Check sheet for the modelled part. Datum: model origin and axes. Units: mm. A direction names the side the tool comes from. Coordinates: 2 decimals unless noted, no trailing zeros. Write each loop counter-clockwise with the first axis right and the second up, starting at its lowest first coordinate (ties: lowest second). Pieces come first, ordered by that corner, then holes. Notation, with made-up numbers: (-10.5, -30) -> (12.5, -30) arc R22 cw to (12.5, 4) -> close; hole circle Ø8 at (-36.75, 9.25). An arc over 180 degrees is marked (long way). One line per item, written item: value. Start each with the question number.
1) Draft check along X on faces 4 (the conical face through (0.621, -0.153, 6.587)), 5 (the flat face through (1, -6, 3)), 6 (the flat face through (3.9, -6, 3)), 7 (the flat face through (4.9, -6, 2)). Enter one of: +X half, -X half, draft (parallel to the pull), parting line (faces both ways), or undercut.
2) Gauge pin test, flat ends, axial feed: P1, Ø2.5, axis at x = 2.5, y = -6, coming from the +Z side; P2, Ø1, axis at x = 3, z = 4.5, coming from the -Y side. Record the tip position at first contact, or that the pin passes through.
3) Sectioned sample at A-A on z = 3. Enter the section's corners in (x, y).
4) Sectioned sample at C-C on x = 2.95. Enter the section's corners in (y, z).
5) Scan lines: line 1 along X through (y, z) = (-5.25, 2.5); line 2 along Z through (x, y) = (1.4, -6.25) (3 decimals); line 3 along Z through (x, y) = (2.8, -11.25). Record each from-to range of solid material in increasing order. Write a range as [from, to].
6) Set-up check for faces 1 (the flat face through (2, -6, 1)), 2 (the flat face through (4.4, -6.4, 5)), 3 (the cylindrical face through (1.21, -6.41, 6.07)): record each of +Z, -Z, +X, -X, +Y, -Y from which the full face is reachable in a straight line by a thin tool's end or side.
7) Sectioned sample at B-B on y = -7.25. Enter the section's corners in (x, z), plus the area to 3 significant figures.
```python
from build123d import *

# Parameters (mm, degrees)
F1_DEPTH     = 13
F2_T1_DEPTH  = 6.0286731952
F2_T3_DEPTH  = 15.0178646599
F2_T5_DEPTH  = 6.9573463904
F2_T7_DEPTH  = 7.0573463904
F2_T10_ANGLE = 67.461453667
F2_T12_ANGLE = 67.461453667


# Not quite as in the source:
# - a fillet or chamfer that OpenCascade refuses, or shapes differently, is made with other operations: its cross-section is extruded or revolved along the edge and cut away or added


with BuildPart() as f1:
    # F0 (on Front) → F1 (new body)
    with BuildSketch(Plane.XZ):
        with BuildLine():
            Line((0, 5), (0, 0))
            Line((0, 0), (4.9, 0))
            Line((4.9, 0), (4.9, 5))
            Line((4.9, 5), (3.9, 5))
            Line((3.9, 5), (3.9, 1))
            Line((3.9, 1), (1, 1))
            Line((1, 1), (1, 5))
            ThreePointArc((1, 5), (1.2914644914, 6.2462400161), (2.1053955316, 7.2339555569))
            Line((2.1053955316, 7.2339555569), (1.4626079219, 8))
            ThreePointArc((1.4626079219, 8), (0.3851271545, 6.6687736465), (0, 5))
        make_face()
    extrude(amount=F1_DEPTH)

    # F2: chamfer of 0.4 on 9 edges, made by hand

    # F2_s2 → F2_t1 (cut)
    with BuildSketch(Plane.XY.offset(-1.0286731952)):
        Polygon((0, -12.6), (0.4, -13), (0, -13), align=None)
        Polygon((0, -0.4), (0.4, 0), (0, 0), align=None)
    extrude(amount=F2_T1_DEPTH, mode=Mode.SUBTRACT)

    # F2_s4 → F2_t3 (cut)
    with BuildSketch(Plane.XZ.offset(-1.00893233)):
        with BuildLine():
            Line((1.8291984844, 6.9931446867), (1.8536490905, 7.5339752825))
            Line((1.8536490905, 7.5339752825), (2.1053955316, 7.2339555569))
            ThreePointArc((2.1053955316, 7.2339555569), (1.9591897538, 7.1144071406), (1.8291984844, 6.9931446867))
        make_face()
    extrude(amount=F2_T3_DEPTH, mode=Mode.SUBTRACT)

    # F2_s6 → F2_t5 (cut)
    with BuildSketch(Plane.YZ.offset(-1.0286731952)):
        Polygon((-0.4, 0), (0, 0.4), (0, 0), align=None)
        Polygon((-12.6, 0), (-13, 0.4), (-13, 0), align=None)
    extrude(amount=F2_T5_DEPTH, mode=Mode.SUBTRACT)

    # F2_s8 → F2_t7 (cut)
    with BuildSketch(Plane.XY.offset(-1.0286731952)):
        Polygon((4.9, -0.4), (4.5, 0), (4.9, 0), align=None)
        Polygon((4.9, -12.6), (4.5, -13), (4.9, -13), align=None)
    extrude(amount=F2_T7_DEPTH, mode=Mode.SUBTRACT)

    # F2_s9 → F2_t10 (revolve, cut)
    with BuildSketch(Plane(origin=(5.0186624957, 0, 2.0827548228), x_dir=(0, 1, 0), z_dir=(0.9236218692, 0, 0.3833048953))):
        Polygon((-0.4, 6.9664843046), (0, 6.5664843046), (0, 6.9664843046), align=None)
    revolve(axis=Axis((3.808, 0, 5), (0, -1, 0)), revolution_arc=F2_T10_ANGLE, mode=Mode.SUBTRACT)

    # F2_s11 → F2_t12 (revolve, cut)
    with BuildSketch(Plane(origin=(5.0186624957, 0, 2.0827548228), x_dir=(0, 1, 0), z_dir=(0.9236218692, 0, 0.3833048953))):
        Polygon((-12.6, 6.9664843046), (-13, 6.5664843046), (-13, 6.9664843046), align=None)
    revolve(axis=Axis((3.808, -13, 5), (0, -1, 0)), revolution_arc=F2_T12_ANGLE, mode=Mode.SUBTRACT)


solid = f1.part
```
Answers:
1. face 4: -X half
1. face 5: undercut
1. face 6: undercut
1. face 7: +X half
2. P1: stops at z = 8
2. P2: passes through
3. outline: (0, -12.6) -> (0.4, -13) -> (1, -13) -> (1, 0) -> (0.4, 0) -> (0, -0.4) -> close; (3.9, -13) -> (4.5, -13) -> (4.9, -12.6) -> (4.9, -0.4) -> (4.5, 0) -> (3.9, 0) -> close
4. outline: (-13, 0.4) -> (-12.6, 0) -> (-0.4, 0) -> (0, 0.4) -> (0, 1) -> (-13, 1) -> close
5. line 1: x = [0, 1], [3.9, 4.9]
5. line 2: z = [0, 1], [6.445, 7.95]
5. line 3: z = [0, 1]
6. face 1: +Y, -Y
6. face 2: +Z, +X, +Y, -Y
6. face 3: +X, +Y, -Y
7. outline: (0, 0) -> (4.9, 0) -> (4.9, 5) -> (3.9, 5) -> (3.9, 1) -> (1, 1) -> (1, 5) arc R2.81 cw to (1.83, 6.99) -> (1.85, 7.53) -> (1.46, 8) arc R3.81 ccw to (0, 5) -> close
7. area: 15.8 mm2
